from build123d import *

# Parameters (mm, degrees)
SKETCH1_R           = 22.5
SKETCH1_R_2         = 2
BOSS_EXTRUDE1_DEPTH = 5
SKETCH2_R           = 4.25
CUT_EXTRUDE1_DEPTH  = 1.5


with BuildPart() as part:
    # Sketch1 → Boss-Extrude1 (new body)
    with BuildSketch(Plane(origin=(0, 0, 0), x_dir=(1, 0, 0), z_dir=(0, 1, 0))):
        with Locations(Location((0, 0, 0), (0, 0, 270))):
            Circle(SKETCH1_R)
        with Locations(Location((0, 15.5, 0), (0, 0, 270))):
            Circle(SKETCH1_R_2, mode=Mode.SUBTRACT)
        with Locations(Location((15.5, 0, 0), (0, 0, 270))):
            Circle(SKETCH1_R_2, mode=Mode.SUBTRACT)
        with Locations(Location((0, -15.5, 0), (0, 0, 270))):
            Circle(SKETCH1_R_2, mode=Mode.SUBTRACT)
        with Locations(Location((-15.5, 0, 0), (0, 0, 270))):
            Circle(SKETCH1_R_2, mode=Mode.SUBTRACT)
        Polygon((7.505553499, 0), (3.75277675, 6.5), (-3.75277675, 6.5), (-7.505553499, 0), (-3.75277675, -6.5), (3.75277675, -6.5), align=None, mode=Mode.SUBTRACT)
    extrude(amount=BOSS_EXTRUDE1_DEPTH)

    # Sketch2 → Cut-Extrude1 (cut)
    with BuildSketch(Plane(origin=(0, 5, 0), x_dir=(1, 0, 0), z_dir=(0, 1, 0))):
        with Locations(Location((0, 15.5, 0), (0, 0, 270))):
            Circle(SKETCH2_R)
        with Locations(Location((15.5, 0, 0), (0, 0, 270))):
            Circle(SKETCH2_R)
        with Locations(Location((0, -15.5, 0), (0, 0, 270))):
            Circle(SKETCH2_R)
        with Locations(Location((-15.5, 0, 0), (0, 0, 270))):
            Circle(SKETCH2_R)
    extrude(amount=-CUT_EXTRUDE1_DEPTH, mode=Mode.SUBTRACT)


solid = part.part
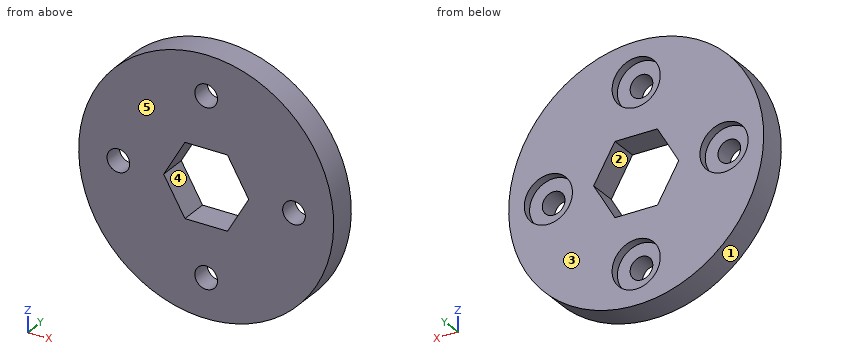
Work out the finished part from the listing and answer in its coordinate system (mm). Face numbers are marked on the shaded views. A direction names the side the tool comes from. Give positions to 0.01 mm unless a question says otherwise; leave off trailing zeros. Order: outer loops, then holes, each group sorted by start corner. A loop starts at its lowest first (then second) coordinate and runs counter-clockwise, first axis right, second up. Notation, with made-up numbers: (3.25, -15.75) - (44.25, -15.75) arc R18 cw to (44.25, -10.75) - close; hole circle Ø9 at (-8, -17). An arc over 180 degrees is marked (long way). Answer as CSV lines item,"result". Start each with the question number.
Q1. For the marked faces 4 and 5, determine the directions among +Z, -Z, +X, -X, +Y, -Y from which every point of the face is accessible in a straight line to the end or side of a thin tool.
Q2. The mould has two halves that part along X. Classify the marked faces 1, 2 and 3: +X half, -X half, draft (parallel to the pull), parting line (faces both ways), or undercut.
Q3. Find the intervals of material crossed by L1, parallel to X at y = 4.15, z = 0; L2, parallel to X at y = 2.3, z = 0; L3, parallel to Z at x = 1.5, y = 1.2, in increasing order. Write a range as [from, to].
Q4. The part is cut by section B-B (x = 0). Write down the section's boundary in (y, z).
Q5. The part is cut by section A-A (y = 1.4). Write down the section's boundary in (x, z).
Q6. Given pin 1 Ø1.5 at (y, z) = (4, 13.5) entering from -X; pin 2 Ø3 at (x, z) = (0, -15.5) entering from +Y; pin 3 Ø10 at (x, z) = (0, -15.5) entering from -Y; pin 4 Ø2.5 at (x, z) = (0, -16.5) entering from +Y, each flat-ended and moving along its own axis, determine where each tip first touches the part or whether it passes through.
Q7. The part is cut by section C-C (z = -15.5). Write down the section's boundary in (x, y).
Q8. The part is cut by section D-D (y = 4.1). Write down the section's boundary in (x, z), then the cut area to 3 significant figures.
Check result:
1,face 4,"+Y, -Y"
1,face 5,"+Z, -Z, +X, -X, -Y"
2,face 1,"parting line"
2,face 2,"undercut"
2,face 3,"draft"
3,L1,"x = [-22.5, -19.75], [-11.25, -7.51], [7.51, 11.25], [19.75, 22.5]"
3,L2,"x = [-22.5, -17.5], [-13.5, -7.51], [7.51, 13.5], [17.5, 22.5]"
3,L3,"z = [-22.45, -16.82], [-14.18, -6.5], [6.5, 14.18], [16.82, 22.45]"
4,outline,"(0, -22.5) - (5, -22.5) - (5, -19.75) - (3.5, -19.75) - (3.5, -17.5) - (0, -17.5) - close; (0, -13.5) - (3.5, -13.5) - (3.5, -11.25) - (5, -11.25) - (5, -6.5) - (0, -6.5) - close; (0, 6.5) - (5, 6.5) - (5, 11.25) - (3.5, 11.25) - (3.5, 13.5) - (0, 13.5) - close; (0, 17.5) - (3.5, 17.5) - (3.5, 19.75) - (5, 19.75) - (5, 22.5) - (0, 22.5) - close"
5,outline,"circle Ø45 at (0, 0); hole circle Ø4 at (-15.5, 0); hole (-7.51, 0) - (-3.75, -6.5) - (3.75, -6.5) - (7.51, 0) - (3.75, 6.5) - (-3.75, 6.5) - close; hole circle Ø4 at (0, -15.5); hole circle Ø4 at (0, 15.5); hole circle Ø4 at (15.5, 0)"
6,pin 1,"stops at x = -18.54"
6,pin 2,"passes through"
6,pin 3,"stops at y = 0"
6,pin 4,"stops at y = 3.5"
7,outline,"(-16.31, 0) - (-2, 0) - (-2, 3.5) - (-4.25, 3.5) - (-4.25, 5) - (-16.31, 5) - close; (2, 0) - (16.31, 0) - (16.31, 5) - (4.25, 5) - (4.25, 3.5) - (2, 3.5) - close"
8,outline,"circle Ø45 at (0, 0); hole circle Ø8.5 at (-15.5, 0); hole (-7.51, 0) - (-3.75, -6.5) - (3.75, -6.5) - (7.51, 0) - (3.75, 6.5) - (-3.75, 6.5) - close; hole circle Ø8.5 at (0, -15.5); hole circle Ø8.5 at (0, 15.5); hole circle Ø8.5 at (15.5, 0)"
8,area,"1,220 mm²"
